Build history of the part. All positions in model axes, mm. A direction names the side the tool comes from. Round coordinates to 2 decimals unless told otherwise and drop trailing zeros. Loops run counter-clockwise (first coordinate to the right, second up) from the corner with the lowest first, then second, coordinate; pieces in that order, holes last. Notation, with made-up numbers: M 58,17 L 69,17 A30 ccw 69,52 Z; hole C 65.5,-19 d1. An arc over 180 degrees is marked long. Use one line per item in the form item = value. Start each with the question number.
```python
from build123d import *

# Parameters (mm, degrees)
BOSS_EXTRUDE1_DEPTH = 3
SKETCH2_R           = 11.1
BOSS_EXTRUDE2_DEPTH = 18
SKETCH3_R           = 9.6
CUT_EXTRUDE1_DEPTH  = 17
FILLET1_R           = 2
SKETCH4_W           = 10
SKETCH4_H           = 6
SKETCH4_W_2         = 6
SKETCH4_H_2         = 18
CUT_EXTRUDE2_DEPTH  = 14
SKETCH5_R           = 4
CUT_EXTRUDE3_DEPTH  = 4
CUT_EXTRUDE4_REACH  = 5
SKETCH6_R           = 1.5
SKETCH7_W           = 5
SKETCH7_H           = 7
BOSS_EXTRUDE3_DEPTH = 23
FILLET2_R           = 2


with BuildPart() as part:
    # Sketch1 → Boss-Extrude1 (new body)
    with BuildSketch(Plane(origin=(0, 5.44100589, 0), x_dir=(-0.502299233, 0, -0.864693865), z_dir=(0, 1, 0))):
        with BuildLine():
            Line((-182.040025286, -110.769690041), (-135.087148398, -138.044538379))
            ThreePointArc((-135.087148398, -138.044538379), (-134.328597463, -138.146454603), (-133.720155299, -137.682143746))
            Line((-133.720155299, -137.682143746), (-106.595996731, -90.988675017))
            ThreePointArc((-106.595996731, -90.988675017), (-106.494080507, -90.230124082), (-106.958391364, -89.621681919))
            Line((-106.958391364, -89.621681919), (-153.911268252, -62.346833581))
            ThreePointArc((-153.911268252, -62.346833581), (-154.669819187, -62.244917357), (-155.27826135, -62.709228213))
            Line((-155.27826135, -62.709228213), (-182.402419919, -109.402696943))
            ThreePointArc((-182.402419919, -109.402696943), (-182.504336143, -110.161247877), (-182.040025286, -110.769690041))
        make_face()
    extrude(amount=BOSS_EXTRUDE1_DEPTH)

    # Sketch2 → Boss-Extrude2 (add)
    with BuildSketch(Plane(origin=(0, 8.44100589, 0), x_dir=(1, 0, 0), z_dir=(0, 1, 0))):
        with Locations((151.220436476, -66.469362794)):
            Circle(SKETCH2_R)
    extrude(amount=BOSS_EXTRUDE2_DEPTH)

    # Sketch3 → Cut-Extrude1 (cut)
    with BuildSketch(Plane(origin=(0, 26.44100589, 0), x_dir=(1, 0, 0), z_dir=(0, 1, 0))):
        with Locations((151.220436476, -66.469362794)):
            Circle(SKETCH3_R)
    extrude(amount=-CUT_EXTRUDE1_DEPTH, mode=Mode.SUBTRACT)

    # Fillet1
    fillet1_edges = [part.edges().sort_by_distance(p)[0] for p in [
        (140.120436476, 8.44100589, 66.469362794),
    ]]
    fillet(fillet1_edges, radius=FILLET1_R)

    # Sketch4 → Cut-Extrude2 (cut)
    with BuildSketch(Plane(origin=(0, 26.44100589, 0), x_dir=(1, 0, 0), z_dir=(0, 1, 0))):
        with Locations((161.220436476, -66.469362794)):
            Rectangle(SKETCH4_W, SKETCH4_H)
        with Locations((151.220436476, -61.469362794)):
            Rectangle(SKETCH4_W_2, SKETCH4_H_2)
    extrude(amount=-CUT_EXTRUDE2_DEPTH, mode=Mode.SUBTRACT)

    # Sketch5 → Cut-Extrude3 (cut)
    with BuildSketch(Plane(origin=(0, 8.44100589, 0), x_dir=(1, 0, 0), z_dir=(0, 1, 0))):
        with Locations((169.220436476, -92.769362794)):
            Circle(SKETCH5_R)
    extrude(amount=-CUT_EXTRUDE3_DEPTH, mode=Mode.SUBTRACT)

    # Sketch6 → Cut-Extrude4 (cut, up to next)
    with BuildSketch(Plane(origin=(0, 8.44100589, 0), x_dir=(1, 0, 0), z_dir=(0, 1, 0)), mode=Mode.PRIVATE) as cut_extrude4_sk1:
        with Locations((179.720436476, -54.469362794)):
            Circle(SKETCH6_R)
    cut_extrude4_tool1 = extrude(cut_extrude4_sk1.sketch, amount=-CUT_EXTRUDE4_REACH, mode=Mode.PRIVATE) & part.part
    add(cut_extrude4_tool1.solids().sort_by_distance((179.720436, 8.441006, 54.469363))[0], mode=Mode.SUBTRACT)
    # Sketch6 → Cut-Extrude4 (cut, up to next)
    with BuildSketch(Plane(origin=(0, 8.44100589, 0), x_dir=(1, 0, 0), z_dir=(0, 1, 0)), mode=Mode.PRIVATE) as cut_extrude4_sk2:
        with Locations((179.720436476, -94.769362794)):
            Circle(SKETCH6_R)
    cut_extrude4_tool2 = extrude(cut_extrude4_sk2.sketch, amount=-CUT_EXTRUDE4_REACH, mode=Mode.PRIVATE) & part.part
    add(cut_extrude4_tool2.solids().sort_by_distance((179.720436, 8.441006, 94.769363))[0], mode=Mode.SUBTRACT)
    # Sketch6 → Cut-Extrude4 (cut, up to next)
    with BuildSketch(Plane(origin=(0, 8.44100589, 0), x_dir=(1, 0, 0), z_dir=(0, 1, 0)), mode=Mode.PRIVATE) as cut_extrude4_sk3:
        with Locations((138.952841808, -95.003108927)):
            Circle(SKETCH6_R)
    cut_extrude4_tool3 = extrude(cut_extrude4_sk3.sketch, amount=-CUT_EXTRUDE4_REACH, mode=Mode.PRIVATE) & part.part
    add(cut_extrude4_tool3.solids().sort_by_distance((138.952842, 8.441006, 95.003109))[0], mode=Mode.SUBTRACT)

    # Sketch7 → Boss-Extrude3 (add)
    with BuildSketch(Plane(origin=(0, 8.44100589, 0), x_dir=(1, 0, 0), z_dir=(0, 1, 0))):
        with Locations((154.220436476, -92.269362794)):
            Rectangle(SKETCH7_W, SKETCH7_H)
    extrude(amount=BOSS_EXTRUDE3_DEPTH)

    # Fillet2
    fillet2_edges = [part.edges().sort_by_distance(p)[0] for p in [
        (156.720436476, 8.44100589, 92.269362794),
        (154.220436476, 8.44100589, 88.769362794),
        (151.720436476, 8.44100589, 92.269362794),
        (154.220436476, 8.44100589, 95.769362794),
    ]]
    fillet(fillet2_edges, radius=FILLET2_R)


solid = part.part
```
Q1. Tool access for faces 1 (the face through (148.814, 18.329, 77.305)), 2 (the face through (157.59, 8.79, 92.19)), 3 (the face through (151.72, 21, 92)), 4 (the face through (154, 21, 95.769)), 5 (the face through (154, 21, 88.769)): list every direction of +Z, -Z, +X, -X, +Y, -Y with a clear straight run to the whole face (end or side of a thin tool).
Q2. Wall check: probe 1 along Y at (x, z) = (162, 57.5); probe 2 along Z at (x, y) = (153.5, 12); probe 3 along X at (y, z) = (7.25, 96). Give the ranges that are in metal, low to high.
Q3. Saw through at D-D (y = 11.25). Give the cut face in (x, z).
Q4. Saw through at B-B (z = 91). Give the cut face in (x, y), and give its area (3 significant figures).
Q5. Saw through at A-A (y = 23.25). Give the cut face in (x, z).
Q6. Pull direction Z, two halves, no side cores. Call faces 6 (the face through (151, 12.441, 56)), 7 (the face through (154.28, 8.79, 96.64)), 8 (the face through (151, 9.441, 66)): pulls with the +Z half, pulls with the -Z half, needs draft (parallel to the pull), parting line crosses it, or undercut.
Q7. Drop flat-ended pins along their axis: P1, Ø2, axis at y = 19.5, z = 93.5, coming from the -X side; P2, Ø3, axis at x = 138.5, z = 68.5, coming from the +Y side; P3, Ø1, axis at x = 161, z = 65, coming from the +Y side. Give the stop position or say it passes through.
Q8. Saw through at C-C (x = 170.5). Give the cut face in (y, z), and give its area (3 significant figures).
Filled in:
q1.face_1 = +Y
q1.face_2 = +Z, +X, +Y
q1.face_3 = +Z, -X, +Y
q1.face_4 = +Z, +X, -X, +Y
q1.face_5 = +X, -X, +Y
q2.probe_1 = 5.44 to 8.44
q2.probe_2 = 55.61 to 57.14, 75.79 to 77.33, 88.77 to 95.77
q2.probe_3 = 131.22 to 137.83, 140.07 to 166.86, 171.58 to 178.86, 180.58 to 187.22
q3.outline = C 151.22,66.47 d22.2; M 151.72,88.77 L 156.72,88.77 L 156.72,95.77 L 151.72,95.77 Z; hole C 151.22,66.47 d19.2
q4.outline = M 131.22,5.44 L 165.63,5.44 L 165.63,8.44 L 158.72,8.44 A2 cw 156.72,10.44 L 156.72,31.44 L 151.72,31.44 L 151.72,10.44 A2 cw 149.72,8.44 L 131.22,8.44 Z; M 172.81,5.44 L 187.22,5.44 L 187.22,8.44 L 172.81,8.44 Z
q4.area = 263 mm²
q5.outline = M 148.22,55.78 L 148.22,57.35 A9.6 cw long 160.34,69.47 L 161.91,69.47 A11.1 ccw long Z; M 151.72,88.77 L 156.72,88.77 L 156.72,95.77 L 151.72,95.77 Z; M 154.22,55.78 A11.1 ccw 161.91,63.47 L 160.34,63.47 A9.6 cw 154.22,57.35 Z
q6.face_6 = needs draft
q6.face_7 = pulls with the +Z half
q6.face_8 = undercut
q7.P1 = 151.72
q7.P2 = 9.42
q7.P3 = 12.44
q8.outline = M 5.44,46.47 L 8.44,46.47 L 8.44,88.98 L 5.44,88.98 Z; M 5.44,96.56 L 8.44,96.56 L 8.44,102.77 L 5.44,102.77 Z
q8.area = 146 mm²
